```python
from build123d import *

# Parameters (mm, degrees)
F0_W     = 54
F0_H     = 24
F1_DEPTH = 2
F2_W     = 48
F2_H     = 18
F3_DEPTH = 5
F4_R     = 0.5


with BuildPart() as f1:
    # F0 (on Top) → F1 (new body)
    with BuildSketch(Plane.XY):
        with Locations((-40.409996, 30.125001)):
            Rectangle(F0_W, F0_H)
    extrude(amount=F1_DEPTH)

    # F2 (on face) → F3 (join)
    with BuildSketch(Plane.XY.offset(2)):
        with Locations((-40.409996, 30.125001)):
            Rectangle(F2_W, F2_H)
    extrude(amount=F3_DEPTH)

    # F4
    f4_edges = [f1.edges().sort_by_distance(p)[0] for p in [
        (-40.409996, 39.125001, 2),
        (-40.409996, 39.125001, 7),
        (-64.409996, 39.125001, 4.5),
        (-16.409996, 30.125001, 2),
        (-16.409996, 30.125001, 7),
        (-40.409996, 21.125001, 7),
        (-40.409996, 21.125001, 2),
        (-64.409996, 30.125001, 7),
        (-64.409996, 30.125001, 2),
        (-64.409996, 21.125001, 4.5),
        (-16.409996, 21.125001, 4.5),
        (-16.409996, 39.125001, 4.5),
        (-13.409996, 30.125001, 2),
        (-13.409996, 30.125001, 0),
        (-13.409996, 18.125001, 1),
        (-40.409996, 18.125001, 0),
        (-40.409996, 18.125001, 2),
        (-67.409996, 30.125001, 2),
        (-67.409996, 18.125001, 1),
        (-67.409996, 30.125001, 0),
        (-67.409996, 42.125001, 1),
        (-40.409996, 42.125001, 2),
        (-40.409996, 42.125001, 0),
        (-13.409996, 42.125001, 1),
    ]]
    fillet(f4_edges, radius=F4_R)


solid = f1.part
```
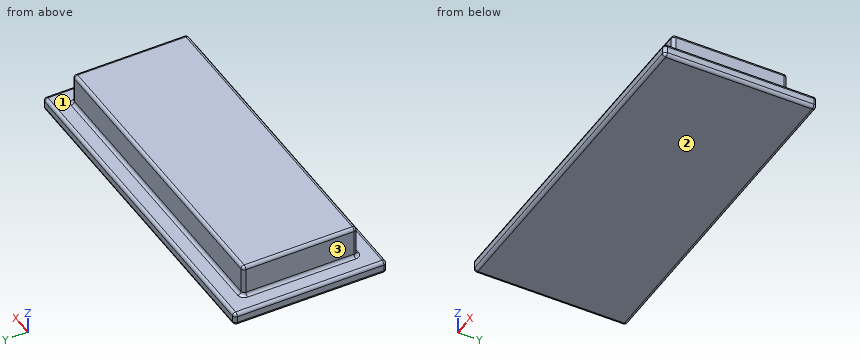
Can you work these out from the model? Positions are in its coordinate system, mm. Face numbers are marked on the shaded views. A direction names the side the tool comes from. Coordinates: 2 decimals unless noted, no trailing zeros. Loops run counter-clockwise (first coordinate to the right, second up) from the corner with the lowest first, then second, coordinate; pieces in that order, holes last. Notation, with made-up numbers: (20.25, 0) -> (39.25, 0) arc R15 ccw to (39.25, 16) -> close; hole circle Ø11 at (-31, 21.25). An arc over 180 degrees is marked (long way). Answer as a JSON object with one key per item and string values.
1) Imagine slicing it at A-A (z = 3.5). Please give me the cut outline in (x, y) (3 decimals).
Results:
{"outline": "(-64.41, 21.625) arc R0.5 ccw to (-63.91, 21.125) -> (-16.91, 21.125) arc R0.5 ccw to (-16.41, 21.625) -> (-16.41, 38.625) arc R0.5 ccw to (-16.91, 39.125) -> (-63.91, 39.125) arc R0.5 ccw to (-64.41, 38.625) -> close"}
2) For the marked faces 1, 2 and 3, which set-ups out of +Z, -Z, +X, -X, +Y, -Y let a thin tool reach every point of the face, with its end or its side?
Results:
{"face 1": "+Z", "face 2": "-Z, +X, -X, +Y, -Y", "face 3": "+Z, -X, +Y, -Y"}
3) For P1, Ø2, axis at x = -49.5, z = 4.5, coming from the +Y side (3 decimals); P2, Ø3, axis at x = -34.5, z = 5, coming from the -Y side (3 decimals); P3, Ø1.5, axis at x = -21.5, z = 2.5, coming from the +Y side, each with a flat end and sliding along its axis, tell me the tip position at first contact or that it passes through.
Results:
{"P1": "stops at y = 39.125", "P2": "stops at y = 21.125", "P3": "stops at y = 42.06"}
4) If I drill on line 1 (X direction, y = 31.25, z = 3); line 2 (Y direction, x = -29.5, z = 2.75) (3 decimals); line 3 (Z direction, x = -64, y = 19.75), over which ranges is the centre line in solid material (lowest first)?
Results:
{"line 1": "x = -64.41 to -16.41", "line 2": "y = 21.125 to 39.125", "line 3": "z = 0 to 2"}
5) Imagine slicing it at B-B (x = -34). Please give me the cut outline in (y, z) (3 decimals).
Results:
{"outline": "(18.125, 0.5) arc R0.5 ccw to (18.625, 0) -> (41.625, 0) arc R0.5 ccw to (42.125, 0.5) -> (42.125, 1.5) arc R0.5 ccw to (41.625, 2) -> (39.625, 2) arc R0.5 cw to (39.125, 2.5) -> (39.125, 6.5) arc R0.5 ccw to (38.625, 7) -> (21.625, 7) arc R0.5 ccw to (21.125, 6.5) -> (21.125, 2.5) arc R0.5 cw to (20.625, 2) -> (18.625, 2) arc R0.5 ccw to (18.125, 1.5) -> close"}
6) Imagine slicing it at C-C (y = 27.75). Please give me the cut outline in (x, z).
Results:
{"outline": "(-67.41, 0.5) arc R0.5 ccw to (-66.91, 0) -> (-13.91, 0) arc R0.5 ccw to (-13.41, 0.5) -> (-13.41, 1.5) arc R0.5 ccw to (-13.91, 2) -> (-15.91, 2) arc R0.5 cw to (-16.41, 2.5) -> (-16.41, 6.5) arc R0.5 ccw to (-16.91, 7) -> (-63.91, 7) arc R0.5 ccw to (-64.41, 6.5) -> (-64.41, 2.5) arc R0.5 cw to (-64.91, 2) -> (-66.91, 2) arc R0.5 ccw to (-67.41, 1.5) -> close"}
